Autodesk Inventor part; units mm, degrees
ref_plane "YZ Plane" through (0, 0, 0) normal (1, 0, 0) x (0, 1, 0)
ref_plane "XZ Plane" through (0, 0, 0) normal (0, 1, 0) x (-1, 0, 0)
ref_plane "XY Plane" through (0, 0, 0) normal (0, 0, 1) x (1, 0, 0)
ref_plane "Work Plane2" through (-6.35, 0, 0) normal (-1, 0, 0) x (0, 0, 1)
ref_plane "Work Plane3" through (0, 0, 0) normal (1, 0, 0) x (0, 0, -1)
sketch "Sketch3" plane through (0, 0, 0) normal (1, 0, 0) x (0, 0, -1)
  circle A0 centre (0, 0) radius 5.08
  dimension "d35" = 10.16
extrude "Extrusion2" add sketch "Sketch3" along normal blind 101.6 and the other way blind 25.4
sketch "Sketch5" plane through (101.6, 0, 0) normal (1, 0, 0) x (0, 0, -1)
  circle A0 centre (0, 0) radius 5.08
ref_plane "Work Plane1" through (-6.35, 0, 18.2681) normal (0, 1, 0) x (1, 0, 0)
sketch "Sketch6" plane through (-6.35, 0, 18.2681) normal (0, 1, 0) x (1, 0, 0)
  point P0 (6.35, 18.2681)
sketch "Sketch7" plane through (-6.35, 0, 18.2681) normal (0, 1, 0) x (1, 0, 0)
  line L0 (107.95, 13.1881) -> (107.95, 23.3481)
  line L1 (107.95, 18.2681) -> (114.3, 18.2681)
  circle A0 centre (114.3, 18.2681) radius 6.35
  circle A1 centre (114.3, 18.2681) radius 9.525
  point P0 (6.35, 18.2681)
  dimension "d50" = 6.35
  dimension "d51" = 19.05
extrude "Extrusion4" add sketch "Sketch7" along normal mid plane 10.16
sketch "Sketch8" plane through (107.95, 5.08, 0) normal (0, 1, 0) x (1, 0, 0)
  point P0 (-107.95, 0)
equation "\"HR\" = 7.874"
equation "\"PR\" = 5.588"
equation "\"HA\" = 55deg"
properties part number "handle with hole"
Input: part model. Units: mm. Frame: model coordinates. A direction names the side the tool comes from. Coordinates: 2 decimals unless noted, no trailing zeros. Loops run counter-clockwise (first coordinate to the right, second up) from the corner with the lowest first, then second, coordinate; pieces in that order, holes last. Notation, with made-up numbers: M 24.5,-4.5 L 28.5,-4.5 A5 ccw 28.5,3.5 Z; hole C -20,-4 d3. An arc over 180 degrees is marked long. Use a Markdown table: item, result. Add a question column.
1) Pin query (flat end, axial travel): P1, Ø2, axis at x = 79.5, z = -4.5, coming from the +Y side; P2, Ø3, axis at x = 92.5, z = 5.5, coming from the +Y side; P3, Ø4, axis at x = 37, y = 2, coming from the +Z side. Return the tip coordinate at first contact, or that it passes through.
2) Section C-C, the plane z = -3. Return the cut outline in (x, y), plus the area to 3 significant figures.
3) Set-up query: faces 1 (the cylindrical face through (38.123, 5.037, 0.661)), 2 (the cylindrical face through (101.606, 0.071, -0.279)). Return all of +Z, -Z, +X, -X, +Y, -Y with unobstructed straight access to the full face (end or side cutting, diameter ignored); none if empty.
4) Section D-D, the plane x = 54. Return the cut outline in (y, z), plus the area to 3 significant figures.
5) Section A-A, the plane x = 107.95. Return the cut outline in (y, z) (3 decimals), plus the area to 3 significant figures.
6) Line query: L1, parallel to Z at x = 107.95, y = -1.5 (3 decimals); L2, parallel to X at y = 2.25, z = 0 (3 decimals); L3, parallel to Z at x = 25, y = 0.5. Output: solid intervals per line, ascending. Write a range as from..to.
7) Section B-B, the plane y = 0. Return the cut outline in (x, z) (3 decimals).
Answer below:
| question | item | result |
|---|---|---|
| 1 | P1 | y = 3.68 |
| 1 | P2 | y = 3.13 |
| 1 | P3 | z = 5.08 |
| 2 | outline | M -25.4,-4.1 L 98.91,-4.1 L 98.91,-5.08 L 102.35,-5.08 L 102.35,5.08 L 98.91,5.08 L 98.91,4.1 L -25.4,4.1 Z; M 113.55,-5.08 L 116.99,-5.08 L 116.99,5.08 L 113.55,5.08 Z |
| 2 | area | 1,090 mm2 |
| 3 | face 1 | -X |
| 3 | face 2 | +Y, -Y |
| 4 | outline | C 0,0 d10.16 |
| 4 | area | 81.1 mm2 |
| 5 | outline | M -5.08,-9.525 L 5.08,-9.525 L 5.08,-6.35 L -5.08,-6.35 Z; M -5.08,6.35 L 5.08,6.35 L 5.08,9.525 L -5.08,9.525 Z |
| 5 | area | 64.5 mm2 |
| 6 | L1 | -9.525..-6.35, 6.35..9.525 |
| 6 | L2 | -25.4..101.6, 114.3..117.475 |
| 6 | L3 | -5.06..5.06 |
| 7 | outline | M -25.4,-5.08 L 99.893,-5.08 A9.525 ccw long 99.893,5.08 L -25.4,5.08 Z; hole C 107.95,0 d12.7 |
